Part model, mm, in its own coordinate system. A direction names the side the tool comes from. Round coordinates to 2 decimals unless told otherwise and drop trailing zeros. Write each loop counter-clockwise with the first axis right and the second up, starting at its lowest first coordinate (ties: lowest second). Pieces come first, ordered by that corner, then holes. Notation, with made-up numbers: M 1,-29 L 59,-29 A16 ccw 59,-4 Z; hole C 76.5,-14 d10. An arc over 180 degrees is marked long. Use a Markdown table: item, result. Add a question column.
1) Slice it at C-C on x = 1.5. Write the cut outline in (y, z) (3 decimals), plus the area to 3 significant figures.
2) Drop flat-ended pins along their axis: P1, Ø0.5, axis at x = 45, z = 5.5, coming from the -Y side; P2, Ø4, axis at y = -12, z = -7, coming from the +X side; P3, Ø4.5, axis at x = 5.5, y = -5.5, coming from the +Z side. Give the stop position or say it passes through.
3) Slice it at D-D on y = -21. Write the cut outline in (x, z) (3 decimals).
4) Which spindle directions (+Z, -Z, +X, -X, +Y, -Y) get a long thin tool onto all of the face, cutting with end or side? Do faces 1 (the face through (42, -37, 5)), 2 (the face through (27.349, -25.868, -8.434)), 3 (the face through (-3.574, 3.605, 4.056)). Say none if no direction does.
5) Slice it at A-A on x = 21. Write the cut outline in (y, z) (3 decimals), plus the area to 3 significant figures.
6) Two-plate mould, pull along Y, no slides. Class faces 4 (the face through (0, -21, 5)), 5 (the face through (21, 0, 5)), 6 (the face through (21, -9, 0)), 7 (the face through (-3.605, -45.574, 4.056)): released by +Y, released by -Y, zero draft, split by the parting line, or undercut.
7) Slice it at B-B on y = -5.5. Write the cut outline in (x, z) (3 decimals), plus the area to 3 significant figures.
8) Wall check: probe 1 along Y at (x, z) = (5.5, 1.6) (3 decimals); probe 2 along X at (y, z) = (-5.5, 1.2) (3 decimals); probe 3 along X at (y, z) = (-7, 6.25) (3 decimals). Give the ranges that are in metal, low to high.
Autodesk Inventor part; units mm, degrees
ref_plane "YZ Plane" through (0, 0, 0) normal (1, 0, 0) x (0, 1, 0)
ref_plane "XZ Plane" through (0, 0, 0) normal (0, 1, 0) x (-1, 0, 0)
ref_plane "XY Plane" through (0, 0, 0) normal (0, 0, 1) x (1, 0, 0)
sketch "Sketch1" plane through (0, 0, 0) normal (0, 0, 1) x (1, 0, 0)
  line L0 (0, 0) -> (42, 0)
  line L1 (42, 0) -> (42, -42)
  line L2 (42, -42) -> (0, -42)
  line L3 (0, -42) -> (0, 0)
  line L4 (0, 0) -> (-1, 0)
  line L5 (-1, 0) -> (-4.175, 0)
  line L6 (-4.175, 0) -> (-4.175, 1)
  line L7 (-4.175, 1) -> (-4.175, 4.175)
  line L8 (-4.175, 4.175) -> (42, 4.175)
  line L9 (42, 4.175) -> (43, 4.175)
  line L10 (43, 4.175) -> (46.175, 4.175)
  line L11 (-4.175, 4.175) -> (46.175, 4.175)
  line L12 (46.175, 4.175) -> (46.175, -46.175)
  line L13 (46.175, -46.175) -> (-4.175, -46.175)
  line L14 (-4.175, -46.175) -> (-4.175, 4.175)
  dimension "d0" = 42
  dimension "d1" = 42
  dimension "d2" = 1
  dimension "d3" = 3.175
  dimension "d4" = 1
  dimension "d5" = 3.175
  dimension "d6" = 1
  dimension "d7" = 3.175
  dimension "d8" = 50.35
extrude "Extrusion1" add sketch "Sketch1" along normal blind 8
sketch "Sketch2" plane through (0, 0, 0) normal (0, 0, -1) x (-1, 0, 0)
  line L0 (0, -42) -> (0, 0)
  line L1 (-42, 0) -> (-42, -42)
  line L2 (0, 0) -> (-42, 0)
  line L3 (-42, 0) -> (-42, -42)
  line L4 (-42, -42) -> (0, -42)
  line L5 (0, -42) -> (0, 0)
extrude "Extrusion2" add sketch "Sketch2" against normal blind 3
sketch "Sketch3" plane through (0, 0, 3) normal (0, 0, 1) x (1, 0, 0)
  line L0 (0, -42) -> (0, 0)
  line L1 (0, -42) -> (21, -42)
  line L2 (42, 0) -> (42, -42)
  line L3 (21, -42) -> (21, -21)
  line L4 (21, -21) -> (21, -36.5)
  line L5 (21, -36.5) -> (36.5, -36.5)
  line L6 (36.5, -36.5) -> (5.5, -36.5)
  line L7 (5.5, -36.5) -> (5.5, -5.5)
  line L8 (5.5, -5.5) -> (36.5, -5.5)
  line L9 (36.5, -5.5) -> (36.5, -36.5)
  dimension "d13" = 21
  dimension "d14" = 21
  dimension "d15" = 15.5
  dimension "d16" = 15.5
  dimension "d17" = 31
  dimension "d18" = 31
hole "Hole1" at (5.5, -5.5, 3) at (36.5, -5.5, 3) at (36.5, -36.5, 3) at (5.5, -36.5, 3) direction (0, 0, -1) diameter 3.5 depth 3.5
sketch "Sketch4" plane through (46.175, -46.175, 0) normal (1, 0, 0) x (0, 0, -1)
  line L0 (0, 0) -> (0, 50.35)
  line L1 (0, 25.175) -> (-3, 25.175)
  line L2 (-3, 46.175) -> (-3, 4.175)
  line L3 (-3, 25.175) -> (-3, 15.175)
  line L4 (-8, 46.175) -> (-8, 4.175)
  line L5 (-3, 15.175) -> (-8, 15.175)
  line L6 (-8, 15.175) -> (-8, 35.175)
  line L7 (-8, 35.175) -> (-3, 35.175)
  line L8 (-3, 35.175) -> (-3, 15.175)
  point P0 (0, 46.175)
  dimension "d26" = 10
  dimension "d27" = 20
extrude "Extrusion3" cut sketch "Sketch4" against normal blind 5
fillet "Fillet1" radius 2 8 edges at (44.0875, -11, 3) (44.0875, -31, 3) (44.0875, -11, 8) (44.0875, -31, 8) (46.175, 4.175, 4) (46.175, -46.175, 4) (-4.175, -46.175, 4) (-4.175, 4.175, 4)
sketch "Sketch5" plane through (0, 0, 3) normal (0, 0, 1) x (1, 0, 0)
  line L0 (42, 0) -> (42, -9)
  line L1 (42, 0) -> (21, 0)
  line L2 (0, 0) -> (42, 0)
  line L3 (21, 0) -> (21, -21)
  dimension "d31" = 21
sketch "Sketch6" plane through (0, 0, 0) normal (0, 0, -1) x (-1, 0, 0)
  line L0 (0, 0) -> (-42, 0)
  line L1 (-21, 0) -> (-21, -21)
  circle A0 centre (-21, -21) radius 11
  dimension "d32" = 21
  dimension "d33" = 22
extrude "Extrusion4" add sketch "Sketch6" along normal blind 11
sketch "Sketch7" plane through (21, -21, -11) normal (0, 0, -1) x (-1, 0, 0)
  circle A0 centre (0, 0) radius 8
  point P0 (21, 21)
  dimension "d36" = 16
extrude "Extrusion5" cut sketch "Sketch7" against normal blind 5
sketch "Sketch8" plane through (21, -21, -6) normal (0, 0, -1) x (-1, 0, 0)
  circle A0 centre (0, 0) radius 5
  point P0 (21, 21)
  dimension "d39" = 10
extrude "Extrusion6" cut sketch "Sketch8" against normal blind 10
fillet "Fillet2" radius 0.2 2 edges at (29, -21, -11) (32, -21, -11)
sketch "Sketch9" plane through (21, -21, -11) normal (0, 0, -1) x (-1, 0, 0)
  line L0 (0, 0) -> (-11, 0)
  circle A0 centre (0, 0) radius 11
  line L1 (-11, 0) -> (-11, -11)
  line L2 (-11, -11) -> (-9, -11)
  line L3 (-9, -11) -> (-9, 11)
  line L4 (-9, 11) -> (-11, 11)
  line L5 (-11, 11) -> (-11, -11)
  point P0 (21, 21)
  dimension "d43" = 11
  dimension "d44" = 2
  dimension "d45" = 22
extrude "Extrusion7" cut sketch "Sketch9" against normal blind 11 contours L3 A0 L0 | L0 A0 L3 | L5 L4 L3 A0 | A0 L3 L2 L1
properties part number "Yaw Shaft Mount"
Entries:
| question | item | result |
|---|---|---|
| 1 | outline | M -46.175,0 L 4.175,0 L 4.175,8 L 0,8 L 0,3 L -42,3 L -42,8 L -46.175,8 Z |
| 1 | area | 193 mm^2 |
| 2 | P1 | stops at y = -46.09 |
| 2 | P2 | stops at x = 29.49 |
| 2 | P3 | stops at z = 3 |
| 3 | outline | M -4.175,0 L 10,0 L 10,-10.8 A0.2 ccw 10.2,-11 L 12.8,-11 A0.2 ccw 13,-10.8 L 13,-6 L 16,-6 L 16,3 L 0,3 L 0,8 L -4.175,8 Z; M 26,-6 L 29,-6 L 29,-10.8 A0.2 ccw 29.2,-11 L 30,-11 L 30,0 L 46.175,0 L 46.175,3 L 26,3 Z |
| 4 | face 1 | +Z |
| 4 | face 2 | -Z |
| 4 | face 3 | +Z, -Z, -X, +Y |
| 5 | outline | M -46.175,0 L -32,0 L -32,-10.8 A0.2 ccw -31.8,-11 L -29.2,-11 A0.2 ccw -29,-10.8 L -29,-6 L -26,-6 L -26,3 L -42,3 L -42,8 L -46.175,8 Z; M -16,-6 L -13,-6 L -13,-10.8 A0.2 ccw -12.8,-11 L -10.2,-11 A0.2 ccw -10,-10.8 L -10,0 L 4.175,0 L 4.175,8 L 0,8 L 0,3 L -16,3 Z |
| 5 | area | 265 mm^2 |
| 6 | face 4 | undercut |
| 6 | face 5 | undercut |
| 6 | face 6 | zero draft |
| 6 | face 7 | released by -Y |
| 7 | outline | M -4.175,0 L 3.75,0 L 3.75,3 L 0,3 L 0,8 L -4.175,8 Z; M 7.25,0 L 34.75,0 L 34.75,3 L 7.25,3 Z; M 38.25,0 L 46.175,0 L 46.175,8 L 42,8 L 42,3 L 38.25,3 Z |
| 7 | area | 172 mm^2 |
| 8 | probe 1 | y = -46.175 to -38.25, -34.75 to -7.25, -3.75 to 4.175 |
| 8 | probe 2 | x = -4.175 to 3.75, 7.25 to 34.75, 38.25 to 46.175 |
| 8 | probe 3 | x = -4.175 to 0, 42 to 46.175 |
